Check sheet for the modelled part. Datum: model origin and axes. Units: mm. Face numbers are marked on the shaded views. A direction names the side the tool comes from. Round coordinates to 2 decimals unless told otherwise and drop trailing zeros. Write each loop counter-clockwise with the first axis right and the second up, starting at its lowest first coordinate (ties: lowest second). Pieces come first, ordered by that corner, then holes.
Item 1: Tool access check on the marked faces 4 and 5. Record the directions out of +Z, -Z, +X, -X, +Y, -Y that give a thin tool (end or side, any length) a straight path to the whole face; none if there is none.
Item 2: Cross-section at B-B on x = -19. Enter the section's corners in (y, z), plus the area to 3 significant figures.
Item 3: Cross-section at A-A on z = 4.4. Enter the section's corners in (x, y), plus the area to 3 significant figures.
Item 4: Cross-section at D-D on x = 17. Enter the section's corners in (y, z), plus the area to 3 significant figures.
Item 5: Go/stop test with flat-tipped pins: pin 1 Ø2 at (y, z) = (0, 2.5) entering from +X; pin 2 Ø1.5 at (y, z) = (0, 2.5) entering from -X. Record where each tip stops, or that it passes through.
Item 6: Material ranges on line 1 (Y direction, x = -28.1, z = 2.5); line 2 (Z direction, x = -28.6, y = -12); line 3 (Y direction, x = -8, z = 3.3), recorded low to high.
Item 7: Cross-section at C-C on y = 0. Enter the section's corners in (x, z), plus the area to 3 significant figures.
Item 8: Release check for a two-part mould opening along Y. For the marked faces 1, 2 and 3 record: +Y half, -Y half, draft (parallel to the pull), parting line (faces both ways), or undercut.
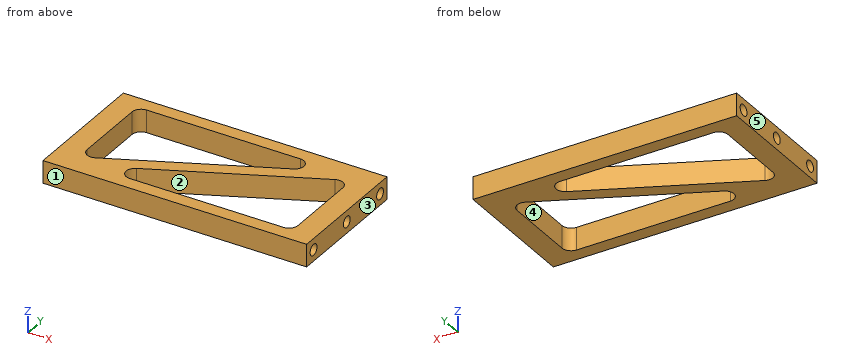
Autodesk Inventor part; units mm, degrees
ref_plane "YZ Plane" through (0, 0, 0) normal (1, 0, 0) x (0, 1, 0)
ref_plane "XZ Plane" through (0, 0, 0) normal (0, 1, 0) x (-1, 0, 0)
ref_plane "XY Plane" through (0, 0, 0) normal (0, 0, 1) x (1, 0, 0)
sketch "スケッチ1" plane through (0, 0, 0) normal (0, 0, 1) x (1, 0, 0)
  line L0 (-29.25, 14.5) -> (29.25, 14.5)
  line L1 (29.25, 14.5) -> (29.25, -14.5)
  line L2 (29.25, -14.5) -> (-29.25, -14.5)
  line L3 (-29.25, -14.5) -> (-29.25, 14.5)
  line L4 (-24.25, 11.5) -> (24.25, 11.5) construction
  line L5 (24.25, 11.5) -> (24.25, -11.5) construction
  line L6 (24.25, -11.5) -> (-24.25, -11.5) construction
  line L7 (-24.25, -11.5) -> (-24.25, 11.5) construction
  line L8 (24.25, 11.5) -> (-24.25, -11.5) construction
  line L9 (-24.25, -9.8399) -> (-24.25, 11.5)
  line L10 (-24.25, 11.5) -> (20.7493, 11.5)
  line L11 (20.7493, 11.5) -> (-24.25, -9.8399)
  line L12 (-20.7493, -11.5) -> (24.25, -11.5)
  line L13 (24.25, -11.5) -> (24.25, 9.8399)
  line L14 (24.25, 9.8399) -> (-20.7493, -11.5)
  line L15 (-29.25, 12) -> (29.25, 12) construction
  line L16 (29.25, -12) -> (-29.25, -12) construction
  line L17 (29.25, 12) -> (29.25, -12) construction
  point P0 (0, 0)
  point P1 (0, 11.5)
  point P2 (0, 14.5)
  point P3 (24.25, 0)
  point P4 (29.25, 0)
  dimension "d0" = 5
  dimension "d1" = 3
  dimension "d2" = 1.5
  dimension "d3" = 24
  dimension "d4" = 2.5
  dimension "d16" = 58.5
extrude "押し出し1" add sketch "スケッチ1" along normal blind 5
sketch "スケッチ2" plane through (29.25, -14.5, 0) normal (1, 0, 0) x (0, 0, -1)
  line L0 (0, 29) -> (-5, 29)
  line L1 (-5, 0) -> (-5, 29)
  line L2 (0, 14.5) -> (-5, 14.5) construction
  point P0 (-2.5, 2.5)
  point P1 (-2.5, 14.5)
  point P2 (-2.5, 26.5)
  point P3 (-2.5, 29)
  dimension "d7" = 24
hole "穴1" at (29.25, -12, 2.5) at (29.25, 0, 2.5) at (29.25, 12, 2.5) direction (-1, 0, 0) diameter 2.459 depth 3
mirror "ミラー1" about plane through (0, 0, 0) normal (1, 0, 0) of "穴1"
fillet "フィレット1" radius 2 6 edges at (-20.7493, -11.5, 2.5) (-24.25, -9.8399, 2.5) (24.25, 9.8399, 2.5) (24.25, -11.5, 2.5) (-24.25, 11.5, 2.5) (20.7493, 11.5, 2.5)
equation "\"d3\" = d5_1"
properties part number "リンク_ふくらはぎ_サブフレーム_1_2(予備案)" material "アルミニウム 2014-T4"
Response values:
1. face 4: +Z, -Z
1. face 5: +Z, -Z, -X, +Y, -Y
2. outline: (-14.5, 0) - (-7.35, 0) - (-7.35, 5) - (-14.5, 5) - close; (11.5, 0) - (14.5, 0) - (14.5, 5) - (11.5, 5) - close
2. area: 50.7 mm2
3. outline: (-29.25, -14.5) - (29.25, -14.5) - (29.25, 14.5) - (-29.25, 14.5) - close; hole (-24.25, -6.68) arc R2 ccw to (-21.39, -8.49) - (12.72, 7.69) arc R2 ccw to (11.86, 11.5) - (-22.25, 11.5) arc R2 ccw to (-24.25, 9.5) - close; hole (-12.72, -7.69) arc R2 ccw to (-11.86, -11.5) - (22.25, -11.5) arc R2 ccw to (24.25, -9.5) - (24.25, 6.68) arc R2 ccw to (21.39, 8.49) - close
3. area: 767 mm2
4. outline: (-14.5, 0) - (-11.5, 0) - (-11.5, 5) - (-14.5, 5) - close; (6.4, 0) - (14.5, 0) - (14.5, 5) - (6.4, 5) - close
4. area: 55.5 mm2
5. pin 1: stops at x = 26.25
5. pin 2: stops at x = -26.25
6. line 1: y = -14.5 to -13.23, -10.77 to -1.23, 1.23 to 10.77, 13.23 to 14.5
6. line 2: z = 0 to 1.27, 3.73 to 5
6. line 3: y = -14.5 to -11.5, -5.45 to -2.13, 11.5 to 14.5
7. outline: (-29.25, 0) - (-24.25, 0) - (-24.25, 5) - (-29.25, 5) - (-29.25, 3.73) - (-26.25, 3.73) - (-26.25, 1.27) - (-29.25, 1.27) - close; (-3.5, 0) - (3.5, 0) - (3.5, 5) - (-3.5, 5) - close; (24.25, 0) - (29.25, 0) - (29.25, 1.27) - (26.25, 1.27) - (26.25, 3.73) - (29.25, 3.73) - (29.25, 5) - (24.25, 5) - close
7. area: 70.3 mm2
8. face 1: -Y half
8. face 2: undercut
8. face 3: draft
